Check sheet for the drawn part. Datum: minimum x, y, z corner. Units: mm. A direction names the side the tool comes from. Give positions to 0.01 mm unless a question says otherwise; leave off trailing zeros. Write each loop counter-clockwise with the first axis right and the second up, starting at its lowest first coordinate (ties: lowest second). Pieces come first, ordered by that corner, then holes. Notation, with made-up numbers: M 17,-15.5 L 66,-15.5 A23 cw 66,13.5 Z; hole C -28,74 d1. An arc over 180 degrees is marked long. Write item = value, one per line.
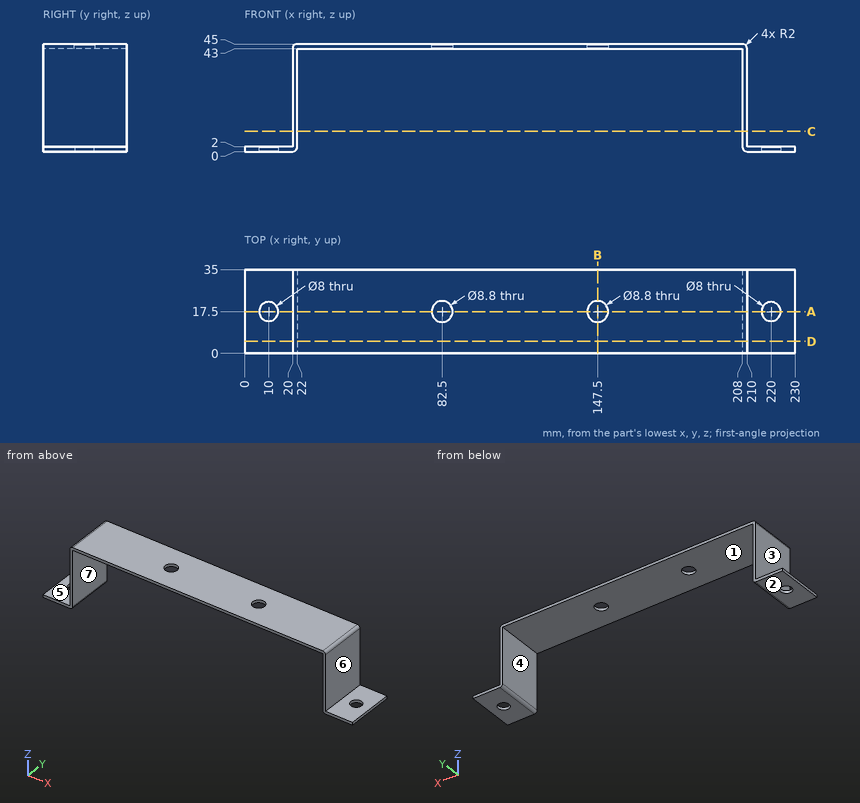
1) Tool access check on the marked faces 5, 6 and 7. Record the directions out of +Z, -Z, +X, -X, +Y, -Y that give a thin tool (end or side, any length) a straight path to the whole face; none if there is none.
From the geometry:
face_5 = +Z, -X, +Y, -Y
face_6 = +Z, +X, +Y, -Y
face_7 = -Z, +Y, -Y
2) Cross-section at C-C on z = 8.5. Record the boundary of the cut face in (x, y).
From the geometry:
outline = M 20,0 L 22,0 L 22,35 L 20,35 Z; M 208,0 L 210,0 L 210,35 L 208,35 Z
3) Cross-section at D-D on y = 5. Record the boundary of the cut face in (x, z), plus the area to 3 significant figures.
From the geometry:
outline = M 0,0 L 20,0 A2 ccw 22,2 L 22,43 L 208,43 L 208,2 A2 ccw 210,0 L 230,0 L 230,2 L 210,2 L 210,43 A2 ccw 208,45 L 22,45 A2 ccw 20,43 L 20,2 L 0,2 Z
area = 629 mm^2
4) Draft check along X on the marked faces 1, 2, 3 and 4. Enter one of: +X half, -X half, draft (parallel to the pull), parting line (faces both ways), or undercut.
From the geometry:
face_1 = undercut
face_2 = draft
face_3 = -X half
face_4 = undercut
5) Cross-section at B-B on x = 147.5. Record the boundary of the cut face in (y, z).
From the geometry:
outline = M 0,43 L 13.1,43 L 13.1,45 L 0,45 Z; M 21.9,43 L 35,43 L 35,45 L 21.9,45 Z
6) Cross-section at A-A on y = 17.5. Count the separate pieces of the cut face and the enclosed holes in it, plus the area to 3 significant figures.
From the geometry:
separate_pieces = 5
enclosed_holes = 0
area = 561 mm^2
7) Depth check by flat-ended pin: P1, Ø6, axis at y = 12.5, z = 4.5, coming from the -X side; P2, Ø1.5, axis at y = 11.5, z = 34.5, coming from the +X side; P3, Ø17.5, axis at x = 80.5, y = 22, coming from the -Z side; P4, Ø6, axis at x = 222, y = 19.5, coming from the +Z side. Enter the tip coordinate at first touch or a pass-through.
From the geometry:
P1 = 0
P2 = 210
P3 = 43
P4 = 2
8) Material ranges on probe 1 along X at (y, z) = (30, 15); probe 2 along Y at (x, z) = (147.5, 44.2); probe 3 along Z at (x, y) = (116, 29), recorded low to high. Write a range as from..to.
From the geometry:
probe_1 = 20..22, 208..210
probe_2 = 0..13.1, 21.9..35
probe_3 = 43..45
